Part model, mm, in its own coordinate system. Face numbers are marked on the shaded views. Round coordinates to 2 decimals unless told otherwise and drop trailing zeros. Order: outer loops, then holes, each group sorted by start corner. A loop starts at its lowest first (then second) coordinate and runs counter-clockwise, first axis right, second up. Notation, with made-up numbers: M 74.25,68 L 98.25,68 A27 cw 98.25,106 Z; hole C 52.5,36.5 d3. An arc over 180 degrees is marked long. Write each question's results on one line, items separated by ' | '. Start each with the question number.
1. Band-saw the part on C-C, the plane y = 0.35. List the corners of the cut face in (x, z) (3 decimals).
2. Two-plate mould, pull along X, no slides. Class the marked faces 1, 2, 3 and 4: +X half, -X half, draft (parallel to the pull), parting line (faces both ways), or undercut.
3. Probe L1, parallel to Z at x = 0, y = 1.95 (3 decimals); L2, parallel to X at y = 0.8, z = 15 (3 decimals); L3, parallel to Z at x = -0.5, y = 1.8. List the from-to ranges inside material, lowest first. Write a range as [from, to].
4. Band-saw the part on A-A, the plane x = 0. List the corners of the cut face in (y, z) (3 decimals), then the cut area to 3 significant figures.
5. Band-saw the part on D-D, the plane x = 2.5. List the corners of the cut face in (y, z).
6. Band-saw the part on B-B, the plane z = 15. List the corners of the cut face in (x, y) (3 decimals), then the cut area to 3 significant figures.
```python
from build123d import *

# Parameters (mm, degrees)
SKETCH_1_W          = 6
SKETCH_1_H          = 40
EXTRUDE_1_DEPTH     = 3
FILLET_1_R          = 2
SKETCH_2_R          = 1.525
CUT_EXTRUDE_1_DEPTH = 3


with BuildPart() as part:
    # 草图1 → 凸台-拉伸1 (new body)
    with BuildSketch(Plane(origin=(0, 0, 0), x_dir=(1, 0, 0), z_dir=(0, 1, 0))):
        Rectangle(SKETCH_1_W, SKETCH_1_H)
    extrude(amount=EXTRUDE_1_DEPTH)

    # 圆角1
    fillet_1_edges = [part.edges().sort_by_distance(p)[0] for p in [
        (3, 1.5, 20),
        (-3, 1.5, 20),
        (-3, 1.5, -20),
        (3, 1.5, -20),
    ]]
    fillet(fillet_1_edges, radius=FILLET_1_R)

    # 草图2 → 切除-拉伸1 (cut)
    with BuildSketch(Plane(origin=(0, 3, 0), x_dir=(1, 0, 0), z_dir=(0, 1, 0))):
        with Locations((0, 5)):
            Circle(SKETCH_2_R)
        with Locations((0, -15)):
            Circle(SKETCH_2_R)
    extrude(amount=-CUT_EXTRUDE_1_DEPTH, mode=Mode.SUBTRACT)


solid = part.part
```
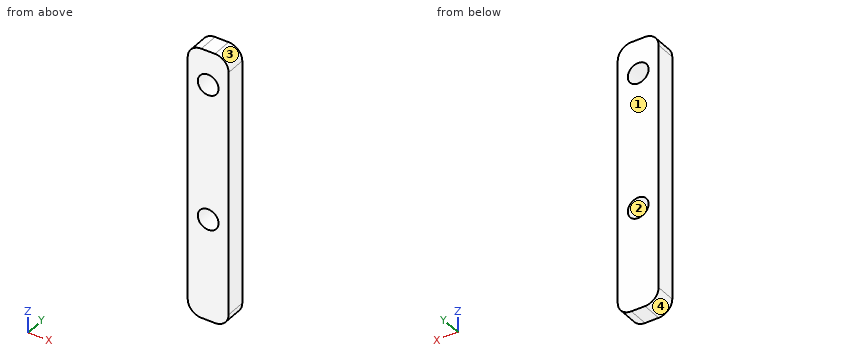
Solution:
1) outline: M -3,-18 A2 ccw -1,-20 L 1,-20 A2 ccw 3,-18 L 3,18 A2 ccw 1,20 L -1,20 A2 ccw -3,18 Z; hole C 0,-5 d3.05; hole C 0,15 d3.05
2) face 1: draft | face 2: undercut | face 3: +X half | face 4: -X half
3) L1: [-20, -6.525], [-3.475, 13.475], [16.525, 20] | L2: [-3, -1.525], [1.525, 3] | L3: [-20, -6.44], [-3.56, 13.56], [16.44, 20]
4) outline: M 0,-20 L 3,-20 L 3,-6.525 L 0,-6.525 Z; M 0,-3.475 L 3,-3.475 L 3,13.475 L 0,13.475 Z; M 0,16.525 L 3,16.525 L 3,20 L 0,20 Z | area: 102 mm^2
5) outline: M 0,-19.32 L 3,-19.32 L 3,19.32 L 0,19.32 Z
6) outline: M -3,0 L -1.525,0 L -1.525,3 L -3,3 Z; M 1.525,0 L 3,0 L 3,3 L 1.525,3 Z | area: 8.85 mm^2
